```python
from build123d import *

# Parameters (mm, degrees)
SKETCH_R        = 16
PAD_DEPTH       = 35
SKETCH001_R     = 14
POCKET_DEPTH    = 23
SKETCH002_R     = 3.98
PAD001_DEPTH    = 10
SKETCH003_W     = 30
SKETCH003_H     = 5.3
POCKET001_DEPTH = 10
SKETCH004_W     = 4.2
SKETCH004_H     = 32.681076
POCKET002_DEPTH = 10


with BuildPart() as part:
    # Sketch → Pad (new body)
    with BuildSketch(Plane.XY):
        Circle(SKETCH_R)
    extrude(amount=PAD_DEPTH)

    # Sketch001 (on Face2 of Pad) → Pocket (cut)
    with BuildSketch(Plane(origin=(0, 0, 0), x_dir=(1, 0, 0), z_dir=(0, 0, -1))):
        Circle(SKETCH001_R)
    extrude(amount=-POCKET_DEPTH, mode=Mode.SUBTRACT)

    # Sketch002 (on Face5 of Pocket) → Pad001 (join)
    with BuildSketch(Plane(origin=(0, 0, 23), x_dir=(1, 0, 0), z_dir=(0, 0, -1))):
        Circle(SKETCH002_R)
    extrude(amount=PAD001_DEPTH)

    # Sketch003 (on Face3 of Pad001) → Pocket001 (cut)
    with BuildSketch(Plane.XY.offset(35)):
        Rectangle(SKETCH003_W, SKETCH003_H)
    extrude(amount=-POCKET001_DEPTH, mode=Mode.SUBTRACT)

    # Sketch004 (on Face3 of Pocket001) → Pocket002 (cut)
    with BuildSketch(Plane.XY.offset(35)):
        with Locations((0, -0.015375)):
            Rectangle(SKETCH004_W, SKETCH004_H)
    extrude(amount=-POCKET002_DEPTH, mode=Mode.SUBTRACT)


solid = part.part
```
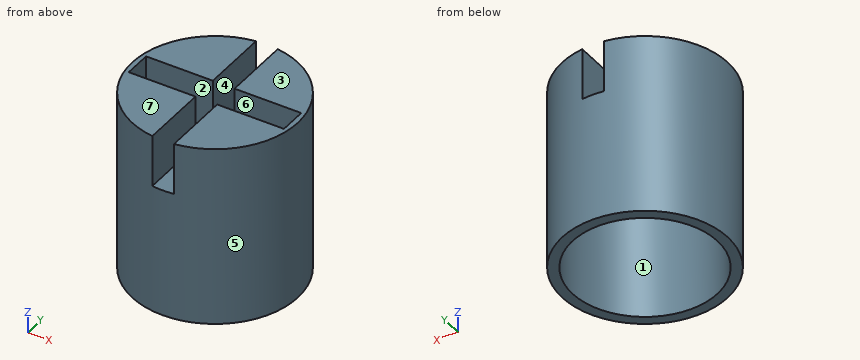
The model under review builds one solid part; all positions refer to its coordinate system, in mm. Face numbers are marked on the shaded views. A direction names the side the tool comes from. Round coordinates to 2 decimals unless told otherwise and drop trailing zeros. Order: outer loops, then holes, each group sorted by start corner. A loop starts at its lowest first (then second) coordinate and runs counter-clockwise, first axis right, second up.
(1) Take a section at C-C, the plane y = 0. State the section outline as (x, z) points.
Working result:
outline: (-16, 0) - (-14, 0) - (-14, 23) - (-3.98, 23) - (-3.98, 13) - (3.98, 13) - (3.98, 23) - (14, 23) - (14, 0) - (16, 0) - (16, 35) - (15, 35) - (15, 25) - (-15, 25) - (-15, 35) - (-16, 35) - close
(2) Take a section at A-A, the plane z = 30. State the section outline as (x, y) points, plus the area to 3 significant figures.
Working result:
outline: (-15, -2.65) - (-15, 2.65) - (-2.1, 2.65) - (-2.1, 15.86) arc R16 ccw to (-2.1, -15.86) - (-2.1, -2.65) - close; (2.1, -15.86) arc R16 ccw to (2.1, 15.86) - (2.1, 2.65) - (15, 2.65) - (15, -2.65) - (2.1, -2.65) - close
area: 533 mm2
(3) For P1, Ø5, axis at y = -9, z = 28.5, coming from the -X side; P2, Ø6.5, axis at x = 2, y = -1, coming from the -Z side; P3, Ø3, axis at x = -9, z = 29.5, coming from the +Y side, all flat-tipped, find the tip position at first contact; note any pin that passes through.
Working result:
P1: stops at x = -14.62
P2: stops at z = 13
P3: stops at y = 14.13
(4) Take a section at D-D, the plane x = 0. State the section outline as (y, z) points, plus the area to 3 significant figures.
Working result:
outline: (-16, 0) - (-14, 0) - (-14, 23) - (-3.98, 23) - (-3.98, 13) - (3.98, 13) - (3.98, 23) - (14, 23) - (14, 0) - (16, 0) - (16, 25) - (-16, 25) - close
area: 236 mm2
(5) Wall thickness on L1, parallel to Y at x = 0, z = 15; L2, parallel to Y at x = 0, z = 6.75; L3, parallel to Y at x = -2, z = 17.5: over which ranges is each line inside the solid? List them lowest first.
Working result:
L1: y = -16 to -14, -3.98 to 3.98, 14 to 16
L2: y = -16 to -14, 14 to 16
L3: y = -15.87 to -13.86, -3.44 to 3.44, 13.86 to 15.87
(6) Mouldability with a two-part tool opening along X and no side actions: class the marked faces 5, 6 and 7 as released by +X, released by -X, zero draft, split by the parting line, or undercut.
Working result:
face 5: split by the parting line
face 6: undercut
face 7: zero draft
(7) Take a section at B-B, the plane z = 14. State the section outline as (x, y) points.
Working result:
outline: circle Ø32 at (0, 0); circle Ø7.96 at (0, 0); hole circle Ø28 at (0, 0)
(8) Tool access review of the marked faces 1, 2, 3 and 4: name each direction out of +Z, -Z, +X, -X, +Y, -Y from which nothing blocks a thin tool from reaching the whole face with its end or side.
Working result:
face 1: -Z
face 2: +Z
face 3: +Z, +X, -X, +Y, -Y
face 4: +Z, +Y, -Y
